Here's the drawing with two shaded views (mm, measured from the low corner). I have some questions. A direction names the side the tool comes from. Give positions to 0.01 mm unless a question says otherwise; leave off trailing zeros. Order: outer loops, then holes, each group sorted by start corner. A loop starts at its lowest first (then second) coordinate and runs counter-clockwise, first axis right, second up. Notation, with made-up numbers: M 16.5,29 L 58.5,29 A13 cw 58.5,52 Z; hole C -15.75,81.5 d6. An arc over 180 degrees is marked long. Use a Markdown table: item, result. Add a question column.
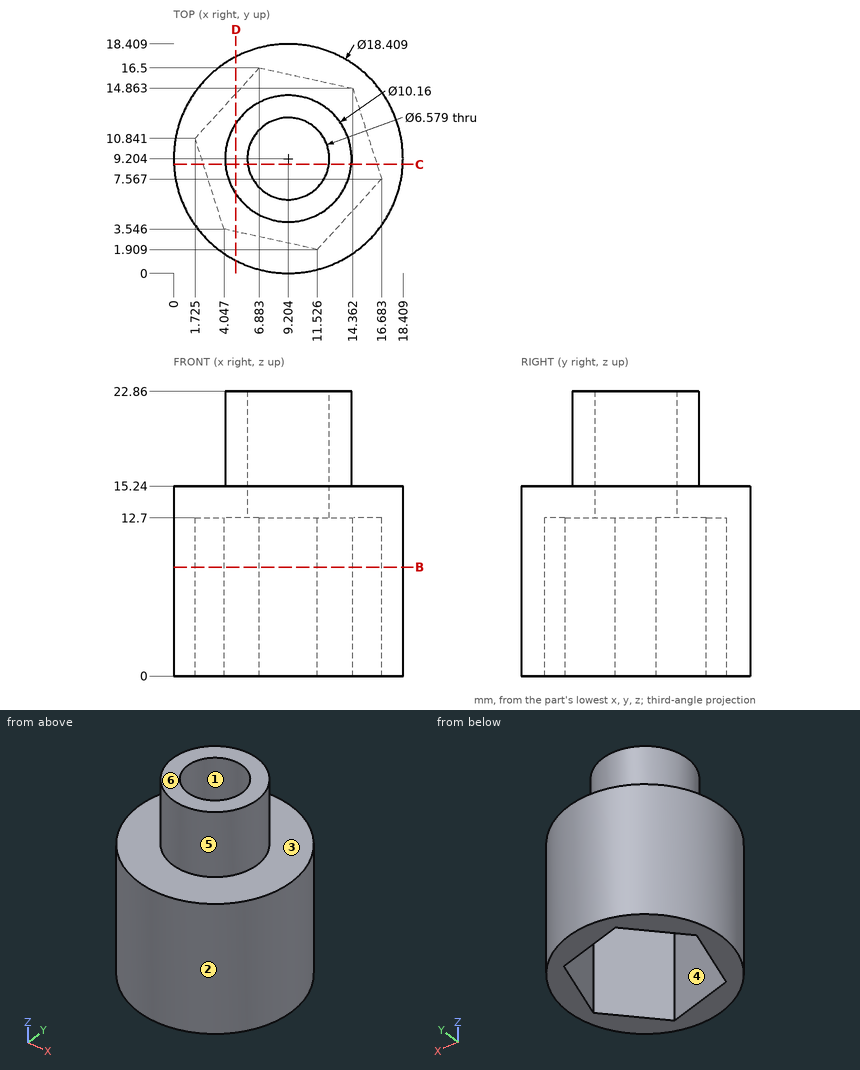
1) Suppose I cut it at D-D on x = 5. Please give me the cut outline in (y, z) (1 decimal), and give its area (3 significant figures).
2) Suppose I cut it at C-C on y = 8.75. Please give me the cut outline in (x, z) (1 decimal).
3) Please list where these lines run through material, in increasing order: line 1 (Z direction, x = 5.75, y = 3.25); line 2 (Z direction, x = 12.5, y = 11.25); line 3 (Y direction, x = 5, z = 4.5) (1 decimal). Write a range as from..to.
4) We'd pull the mould along X, two halves only. Please class the marked faces 1, 2 and 3: pulls with the +X half, pulls with the -X half, needs draft (parallel to the pull), parting line crosses it, or undercut.
5) Suppose I cut it at B-B on z = 8.75. Please give me the cut outline in (x, y) (1 decimal), and give its area (3 significant figures).
6) For the marked faces 4, 5 and 6, which set-ups out of +Z, -Z, +X, -X, +Y, -Y let a thin tool reach every point of the face, with its end or its side?
7) For pin 1 (1 mm diameter, centred on x = 15.5, z = 11, fed in from +Y) (1 decimal); pin 2 (3 mm diameter, centred on x = 11, y = 13.5, fed in from -Z); pin 3 (4 mm diameter, centred on y = 12.5, z = 13, fed in from -X), each with a flat end and sliding along its axis, tell me the tip position at first contact or that it passes through.
Values found:
| question | item | result |
|---|---|---|
| 1 | outline | M 1,0 L 3.3,0 L 3.3,12.7 L 14.4,12.7 L 14.4,0 L 17.4,0 L 17.4,15.2 L 12.1,15.2 L 12.1,22.9 L 6.4,22.9 L 6.4,15.2 L 1,15.2 Z |
| 1 | area | 152 mm^2 |
| 2 | outline | M 0,0 L 2.4,0 L 2.4,12.7 L 5.9,12.7 L 5.9,22.9 L 4.1,22.9 L 4.1,15.2 L 0,15.2 Z; M 12.5,12.7 L 16.3,12.7 L 16.3,0 L 18.4,0 L 18.4,15.2 L 14.3,15.2 L 14.3,22.9 L 12.5,22.9 Z |
| 3 | line 1 | z = 12.7..15.24 |
| 3 | line 2 | z = 12.7..22.86 |
| 3 | line 3 | y = 1..3.3, 14.4..17.4 |
| 4 | face 1 | undercut |
| 4 | face 2 | parting line crosses it |
| 4 | face 3 | needs draft |
| 5 | outline | C 9.2,9.2 d18.4; hole M 1.7,10.8 L 4,3.5 L 11.5,1.9 L 16.7,7.6 L 14.4,14.9 L 6.9,16.5 Z |
| 5 | area | 114 mm^2 |
| 6 | face 4 | -Z |
| 6 | face 5 | +Z |
| 6 | face 6 | +Z, +X, -X, +Y, -Y |
| 7 | pin 1 | stops at y = 16.4 |
| 7 | pin 2 | stops at z = 12.7 |
| 7 | pin 3 | stops at x = 0.09 |
